```python
from build123d import *

# Parameters (mm, degrees)
SKETCH2_R          = 1
CUT_EXTRUDE1_DEPTH = 0.3
CHAMFER1_SIZE      = 0.3
SKETCH3_R          = 1
CUT_EXTRUDE2_DEPTH = 0.7


with BuildPart() as part:
    # Sketch1 → Revolve1 (revolve)
    with BuildSketch(Plane(origin=(0, 0, 0), x_dir=(1, 0, 0), z_dir=(0, 1, 0)), mode=Mode.PRIVATE) as revolve1_sk:
        Polygon((-7, 0), (-7, 2), (-6, 3), (0, 3), (0, 5), (2.8, 5), (8, 1.9977786), (8, 0), align=None)
    revolve(revolve1_sk.sketch.rotate(Axis((-2.427745665, 0, 0), (1, 0, 0)), 180), axis=Axis((-2.427745665, 0, 0), (1, 0, 0)))

    # Sketch2 → Cut-Extrude1 (cut)
    with BuildSketch(Plane(origin=(8, 0, 0), x_dir=(0, 0, -1), z_dir=(1, 0, 0))):
        Circle(SKETCH2_R)
    extrude(amount=-CUT_EXTRUDE1_DEPTH, mode=Mode.SUBTRACT)

    # Chamfer1
    chamfer1_edges = [part.edges().sort_by_distance(p)[0] for p in [
        (8, 0, 1),
    ]]
    chamfer(chamfer1_edges, length=CHAMFER1_SIZE - 0.0001)  # a hair under: the kernel refuses the full size

    # Sketch3 → Cut-Extrude2 (cut)
    with BuildSketch(Plane(origin=(7.7, 0, 0), x_dir=(0, 0, -1), z_dir=(1, 0, 0))):
        Circle(SKETCH3_R)
    extrude(amount=-CUT_EXTRUDE2_DEPTH, mode=Mode.SUBTRACT)

    # Cut-Extrude3 cone 1 section (through the dimple's axis) → Cut-Extrude3 (revolve, cut)
    with BuildSketch(Plane(origin=(7, 0, 0), x_dir=(0, 0, -1), z_dir=(0, 1, 0))):
        Polygon((0, 0), (1, 0), (0, 1), align=None)
    revolve(axis=Axis((7, 0, 0), (-1, 0, 0)), mode=Mode.SUBTRACT)


solid = part.part
```
Source: CAD feature listing. Evaluate the final solid. Frame: model axes, mm. A direction names the side the tool comes from. Coordinates: 2 decimals unless noted, no trailing zeros. Loops run counter-clockwise (first coordinate to the right, second up) from the corner with the lowest first, then second, coordinate; pieces in that order, holes last. Notation, with made-up numbers: (-34, 41) -> (-9, 41) arc R37 ccw to (-9, 80) -> close; hole circle Ø9 at (-19.75, -39). An arc over 180 degrees is marked (long way). One line per item, written item: value. Start each with the question number.
Q1. Set-up query: faces 4 (the face through (-2.96, -0.9, 2.86)), 5 (the face through (7.17, -0.744, 2.363)). Return all of +Z, -Z, +X, -X, +Y, -Y with unobstructed straight access to the full face (end or side cutting, diameter ignored); none if empty.
Q2. Contact query for flat-ended pins moving along their axis: P1, Ø2.5, axis at y = 0, z = 0, coming from the +X side; P2, Ø2, axis at x = 1, z = -1.5, coming from the -Y side; P3, Ø3, axis at x = 5, z = 0.5, coming from the -Y side. Output: stop coordinate, or through.
Q3. Section query A-A, the plane x = 2. Return the cut outline in (y, z).
Q4. Line query: line 1 along Y through (x, z) = (7.5, 0); line 2 along Y through (x, z) = (7.25, 0); line 3 along X through (y, z) = (0.5, -2). Output: solid intervals per line, ascending.
Q5. Mould query, pull axis Z, two halves, no side actions, for faces 1 (the face through (1, 0, -5)), 2 (the face through (7.355, -0.976, 0.217)), 3 (the face through (0, 3.3, 0.1)). Classes: pulls with the +Z half, pulls with the -Z half, needs draft (parallel to the pull), parting line crosses it, or undercut.
Results:
1. face 4: -X
1. face 5: +X
2. P1: x = 7.95
2. P2: y = -4.97
2. P3: y = -4.58
3. outline: circle Ø10 at (0, 0)
4. line 1: -2.29 to -1, 1 to 2.29
4. line 2: -2.43 to -1, 1 to 2.43
4. line 3: -6.94 to 7.89
5. face 1: parting line crosses it
5. face 2: undercut
5. face 3: needs draft
